Geometry: final body of the model. Coordinates: model frame, mm. A direction names the side the tool comes from. Give positions to 0.01 mm unless a question says otherwise; leave off trailing zeros. Write each loop counter-clockwise with the first axis right and the second up, starting at its lowest first coordinate (ties: lowest second). Pieces come first, ordered by that corner, then holes. Notation, with made-up numbers: M 23.25,29.5 L 39.25,29.5 A32 cw 39.25,66.5 Z; hole C 35,14 d6. An arc over 180 degrees is marked long. Use a Markdown table: item, result. Add a question column.
1) Section C-C on z = 2.05. Return the cut outline in (x, y) (3 decimals).
2) Section B-B on y = -1. Return the cut outline in (x, z), then the cut area to 3 significant figures.
3) Pin query (flat end, axial travel): pin 1 (2 mm diameter, centred on x = -13, z = 1.5, fed in from +Y); pin 2 (1.2 mm diameter, centred on y = -6.5, z = 2, fed in from +X) (3 decimals); pin 3 (1.2 mm diameter, centred on y = -6.5, z = 2, fed in from -X) (3 decimals). Return the tip coordinate at first contact, or that it passes through.
4) Section D-D on y = 7. Return the cut outline in (x, z) (3 decimals).
5) Section A-A on x = -14. Return the cut outline in (y, z).
6) Set-up query: faces 1 (the flat face through (-15, -4.608, 2)), 2 (the flat face through (10.375, -8, 2)), 3 (the flat face through (-15, 6.081, 2)), 4 (the flat face through (10.375, 8, 2)). Return all of +Z, -Z, +X, -X, +Y, -Y with unobstructed straight access to the full face (end or side cutting, diameter ignored); none if empty.
7) Draft query along Y for faces 5 (the cylindrical face through (-11.235, 1.732, 1.972)), 6 (the flat face through (19.764, 1, 2)), 7 (the flat face through (0, 10.375, 2)). Return one class per face: +Y half, -Y half, draft (parallel to the pull), parting line (faces both ways), or undercut.
8) Line query: line 1 (X direction, y = 3.5, z = 0.35); line 2 (X direction, y = 1.5, z = 0.3); line 3 (X direction, y = 9, z = 3.45) (3 decimals). Output: solid intervals per line, ascending.
```python
from build123d import *

# Parameters (mm, degrees)
SKETCH1_R           = 3.475
BOSS_EXTRUDE1_DEPTH = 4


with BuildPart() as part:
    # Sketch1 → Boss-Extrude1 (new body)
    # profile 1 of 3: a face of its own
    with BuildSketch(Plane.XY):
        with BuildLine():
            Line((-10.375, 6.080549062), (-19.564197283, 6.080549062))
            ThreePointArc((-19.564197283, 6.080549062), (-19.70561864, 6.021970418), (-19.764197283, 5.880549062))
            Line((-19.764197283, 5.880549062), (-19.764197283, -4.408416131))
            ThreePointArc((-19.764197283, -4.408416131), (-19.70561864, -4.549837487), (-19.564197283, -4.608416131))
            Line((-19.564197283, -4.608416131), (-10.375, -4.608416131))
            Line((-10.375, -4.608416131), (-10.375, 6.080549062))
        make_face()
        with Locations((-14.549223744, 0.688062131)):
            Circle(SKETCH1_R, mode=Mode.SUBTRACT)
    # profile 2 of 3: a face of its own
    with BuildSketch(Plane.XY):
        Polygon((-10.375, 10.375), (-10.375, 6.080549062), (-10.375, -4.608416131), (-10.375, -10.375), (10.375, -10.375), (10.375, -4.608416131), (10.375, 6.080549062), (10.375, 10.375), align=None)
    # profile 3 of 3: a face of its own
    with BuildSketch(Plane.XY):
        with BuildLine():
            Line((19.764197283, 5.880549062), (19.764197283, -4.408416131))
            ThreePointArc((19.764197283, -4.408416131), (19.70561864, -4.549837487), (19.564197283, -4.608416131))
            Line((19.564197283, -4.608416131), (10.375, -4.608416131))
            Line((10.375, -4.608416131), (10.375, 6.080549062))
            Line((10.375, 6.080549062), (19.564197283, 6.080549062))
            ThreePointArc((19.564197283, 6.080549062), (19.70561864, 6.021970418), (19.764197283, 5.880549062))
        make_face()
        with Locations((14.989443539, 0.688062131)):
            Circle(SKETCH1_R, mode=Mode.SUBTRACT)
    extrude(amount=BOSS_EXTRUDE1_DEPTH)


solid = part.part
```
Found:
| question | item | result |
|---|---|---|
| 1 | outline | M -19.764,-4.408 A0.2 ccw -19.564,-4.608 L -10.375,-4.608 L -10.375,-10.375 L 10.375,-10.375 L 10.375,-4.608 L 19.564,-4.608 A0.2 ccw 19.764,-4.408 L 19.764,5.881 A0.2 ccw 19.564,6.081 L 10.375,6.081 L 10.375,10.375 L -10.375,10.375 L -10.375,6.081 L -19.564,6.081 A0.2 ccw -19.764,5.881 Z; hole C -14.549,0.688 d6.95; hole C 14.989,0.688 d6.95 |
| 2 | outline | M -19.76,0 L -17.59,0 L -17.59,4 L -19.76,4 Z; M -11.51,0 L 11.95,0 L 11.95,4 L -11.51,4 Z; M 18.03,0 L 19.76,0 L 19.76,4 L 18.03,4 Z |
| 2 | area | 110 mm² |
| 3 | pin 1 | y = 6.08 |
| 3 | pin 2 | x = 10.375 |
| 3 | pin 3 | x = -10.375 |
| 4 | outline | M -10.375,0 L 10.375,0 L 10.375,4 L -10.375,4 Z |
| 5 | outline | M -4.61,0 L -2.74,0 L -2.74,4 L -4.61,4 Z; M 4.12,0 L 6.08,0 L 6.08,4 L 4.12,4 Z |
| 6 | face 1 | +Z, -Z, -X, -Y |
| 6 | face 2 | +Z, -Z, +X, -Y |
| 6 | face 3 | +Z, -Z, -X, +Y |
| 6 | face 4 | +Z, -Z, +X, +Y |
| 7 | face 5 | undercut |
| 7 | face 6 | draft |
| 7 | face 7 | +Y half |
| 8 | line 1 | -19.76 to -16.59, -12.51 to 12.95, 17.03 to 19.76 |
| 8 | line 2 | -19.76 to -17.93, -11.17 to 11.61, 18.37 to 19.76 |
| 8 | line 3 | -10.375 to 10.375 |
